from build123d import *

# Parameters (mm, degrees)
BOSS_EXTRUDE23_DEPTH = 1
BOSS_EXTRUDE27_DEPTH = 6
BOSS_EXTRUDE28_START = 6
BOSS_EXTRUDE28_DEPTH = 1
CUT_EXTRUDE9_DEPTH   = 1
SKETCH15_W           = 10
SKETCH15_H           = 2
CUT_EXTRUDE11_DEPTH  = 10
BOSS_EXTRUDE30_DEPTH = 4
BOSS_EXTRUDE31_DEPTH = 3


with BuildPart() as part:
    # Sketch10 → Boss-Extrude23 (new body)
    with BuildSketch(Plane(origin=(0, 0, 0), x_dir=(1, 0, 0), z_dir=(0, 1, 0))):
        with BuildLine():
            Line((-11.5, -13.5), (-10.75, -13.5))
            ThreePointArc((-10.75, -13.5), (-10.603553391, -13.853553391), (-10.25, -14))
            Line((-10.25, -14), (10.25, -14))
            ThreePointArc((10.25, -14), (10.603553391, -13.853553391), (10.75, -13.5))
            Line((10.75, -13.5), (11.5, -13.5))
            Line((11.5, -13.5), (11.5, 13.75))
            ThreePointArc((11.5, 13.75), (11.207106781, 14.457106781), (10.5, 14.75))
            Line((10.5, 14.75), (-10.5, 14.75))
            ThreePointArc((-10.5, 14.75), (-11.207106781, 14.457106781), (-11.5, 13.75))
            Line((-11.5, 13.75), (-11.5, -13.5))
        make_face()
    extrude(amount=BOSS_EXTRUDE23_DEPTH)

    # Sketch10_6 → Boss-Extrude27 (add)
    with BuildSketch(Plane(origin=(0, 0, 0), x_dir=(1, 0, 0), z_dir=(0, 1, 0))):
        with BuildLine():
            Line((-11.5, -13.5), (-10.75, -13.5))
            Line((-10.75, -13.5), (-10.75, 13.5))
            ThreePointArc((-10.75, 13.5), (-10.603553391, 13.853553391), (-10.25, 14))
            Line((-10.25, 14), (10.25, 14))
            ThreePointArc((10.25, 14), (10.603553391, 13.853553391), (10.75, 13.5))
            Line((10.75, 13.5), (10.75, -13.5))
            Line((10.75, -13.5), (11.5, -13.5))
            Line((11.5, -13.5), (11.5, 13.75))
            ThreePointArc((11.5, 13.75), (11.207106781, 14.457106781), (10.5, 14.75))
            Line((10.5, 14.75), (4.75, 14.75))
            Line((4.75, 14.75), (-4.75, 14.75))
            Line((-4.75, 14.75), (-10.5, 14.75))
            ThreePointArc((-10.5, 14.75), (-11.207106781, 14.457106781), (-11.5, 13.75))
            Line((-11.5, 13.75), (-11.5, -13.5))
        make_face()
    extrude(amount=BOSS_EXTRUDE27_DEPTH)

    # Sketch10_7 → Boss-Extrude28 (add)
    with BuildSketch(Plane(origin=(0, 0, 0), x_dir=(1, 0, 0), z_dir=(0, 1, 0)).offset(BOSS_EXTRUDE28_START)):
        with BuildLine():
            Line((-11.5, -13.5), (-10.75, -13.5))
            Line((-10.75, -13.5), (-10.75, 13.5))
            ThreePointArc((-10.75, 13.5), (-10.603553391, 13.853553391), (-10.25, 14))
            Line((-10.25, 14), (10.25, 14))
            ThreePointArc((10.25, 14), (10.603553391, 13.853553391), (10.75, 13.5))
            Line((10.75, 13.5), (10.75, -13.5))
            Line((10.75, -13.5), (11.5, -13.5))
            Line((11.5, -13.5), (11.5, 13.75))
            ThreePointArc((11.5, 13.75), (11.207106781, 14.457106781), (10.5, 14.75))
            Line((10.5, 14.75), (4.75, 14.75))
            Line((4.75, 14.75), (-4.75, 14.75))
            Line((-4.75, 14.75), (-10.5, 14.75))
            ThreePointArc((-10.5, 14.75), (-11.207106781, 14.457106781), (-11.5, 13.75))
            Line((-11.5, 13.75), (-11.5, -13.5))
        make_face()
        with BuildLine():
            Line((10.75, 13.5), (10.75, -13.5))
            ThreePointArc((10.75, -13.5), (10.603553391, -13.853553391), (10.25, -14))
            Line((10.25, -14), (-10.25, -14))
            ThreePointArc((-10.25, -14), (-10.603553391, -13.853553391), (-10.75, -13.5))
            Line((-10.75, -13.5), (-10.75, 13.5))
            ThreePointArc((-10.75, 13.5), (-10.603553391, 13.853553391), (-10.25, 14))
            Line((-10.25, 14), (10.25, 14))
            ThreePointArc((10.25, 14), (10.603553391, 13.853553391), (10.75, 13.5))
        make_face()
    extrude(amount=BOSS_EXTRUDE28_DEPTH)

    # Sketch13 → Cut-Extrude9 (cut)
    with BuildSketch(Plane(origin=(0, 7, 0), x_dir=(1, 0, 0), z_dir=(0, 1, 0))):
        with BuildLine():
            Line((-5, -14), (5, -14))
            ThreePointArc((5, -14), (0, -9), (-5, -14))
        make_face()
    extrude(amount=-CUT_EXTRUDE9_DEPTH, mode=Mode.SUBTRACT)

    # Sketch15 → Cut-Extrude11 (cut)
    with BuildSketch(Plane(origin=(0, 0, -14.75), x_dir=(-1, 0, 0), z_dir=(0, 0, -1))):
        with Locations((0, 2)):
            Rectangle(SKETCH15_W, SKETCH15_H)
    extrude(amount=-CUT_EXTRUDE11_DEPTH, mode=Mode.SUBTRACT)

    # Sketch17 → Boss-Extrude30 (add)
    with BuildSketch(Plane(origin=(0, 7, 0), x_dir=(1, 0, 0), z_dir=(0, 1, 0))):
        with BuildLine():
            Line((-9.25, -6.75), (-9.25, 14.75))
            Line((-9.25, 14.75), (-10, 14.75))
            Line((-10, 14.75), (-10, -7))
            ThreePointArc((-10, -7), (-9.707106781, -7.707106781), (-9, -8))
            Line((-9, -8), (9, -8))
            ThreePointArc((9, -8), (9.707106781, -7.707106781), (10, -7))
            Line((10, -7), (10, 14.75))
            Line((10, 14.75), (9.25, 14.75))
            Line((9.25, 14.75), (9.25, -6.75))
            ThreePointArc((9.25, -6.75), (9.103553391, -7.103553391), (8.75, -7.25))
            Line((8.75, -7.25), (-8.75, -7.25))
            ThreePointArc((-8.75, -7.25), (-9.103553391, -7.103553391), (-9.25, -6.75))
        make_face()
    extrude(amount=BOSS_EXTRUDE30_DEPTH)

    # Sketch18 → Boss-Extrude31 (add)
    with BuildSketch(Plane(origin=(0, 7, 0), x_dir=(1, 0, 0), z_dir=(0, 1, 0))):
        with BuildLine():
            Line((9, 7.5), (9.25, 7.5))
            Line((9.25, 7.5), (9.25, 14.75))
            Line((9.25, 14.75), (8, 14.75))
            Line((8, 14.75), (8, 8.5))
            ThreePointArc((8, 8.5), (8.292893219, 7.792893219), (9, 7.5))
        make_face()
        with BuildLine():
            Line((5, -1.656788855), (0, -1.656788855))
            ThreePointArc((0, -1.656788855), (-0.5, -1.156788855), (0, -0.656788855))
            Line((0, -0.656788855), (5, -0.656788855))
            ThreePointArc((5, -0.656788855), (5.5, -1.156788855), (5, -1.656788855))
        make_face()
        with BuildLine():
            Line((-9.25, 7.5), (-9, 7.5))
            ThreePointArc((-9, 7.5), (-8.292893219, 7.792893219), (-8, 8.5))
            Line((-8, 8.5), (-8, 14.75))
            Line((-8, 14.75), (-9.25, 14.75))
            Line((-9.25, 14.75), (-9.25, 7.5))
        make_face()
    extrude(amount=BOSS_EXTRUDE31_DEPTH)


solid = part.part
Read the model definition and answer for the solid it produces. Units are mm, in the model's axes. A direction names the side the tool comes from. Coordinates: 2 decimals unless noted, no trailing zeros. Loops run counter-clockwise (first coordinate to the right, second up) from the corner with the lowest first, then second, coordinate; pieces in that order, holes last. Notation, with made-up numbers: (-12, -27.75) -> (7, -27.75) arc R24 cw to (7, 10.25) -> close; hole circle Ø10 at (67.25, -8). An arc over 180 degrees is marked (long way). Write item = value, one per line. Start each with the question number.
1) Given P1, Ø1, axis at x = -8.5, z = -10.5, coming from the +Y side; P2, Ø4, axis at x = 2.5, y = 4.5, coming from the +Z side; P3, Ø1.5, axis at x = 1.5, y = 9, coming from the -Z side, each flat-ended and moving along its own axis, determine where each tip first touches the part or whether it passes through.
2) Find the intervals of material crossed by L1, parallel to X at y = 3.25, z = -11; L2, parallel to Y at x = 8.5, z = -2.5; L3, parallel to Z at x = 1.5, y = 7.75, in increasing order. Write a range as from..to.
3) The part is cut by section C-C, the plane y = 5.25. Determine the outline of the cut face in (x, z).
4) The mould has two halves that part along Y. Classify faces 1 (the face through (-8.301, 8.479, -7.785)), 2 (the face through (-10.75, 3, 0)), 3 (the face through (-9, 10, -11)): pulls with the +Y half, pulls with the -Y half, needs draft (parallel to the pull), parting line crosses it, or undercut.
5) The part is cut by section A-A, the plane x = 6.25. Determine the outline of the cut face in (y, z).
6) For faces 4 (the face through (9, 10, -11)), 5 (the face through (9.25, 9, -2)), 6 (the face through (0, 9, 8)), determine the directions among +Z, -Z, +X, -X, +Y, -Y from which every point of the face is accessible in a straight line to the end or side of a thin tool.
7) The part is cut by section D-D, the plane x = -4.5. Determine the outline of the cut face in (y, z).
8) The part is cut by section B-B, the plane z = -11.25. Determine the outline of the cut face in (x, y).
Result:
q1.P1 = 10
q1.P2 = 10.78
q1.P3 = 0.66
q2.L1 = -11.5..-10.75, 10.75..11.5
q2.L2 = 0..1, 6..7
q2.L3 = 0.66..1.66, 7.25..8
q3.outline = (-11.5, -13.75) arc R1 ccw to (-10.5, -14.75) -> (10.5, -14.75) arc R1 ccw to (11.5, -13.75) -> (11.5, 13.5) -> (10.75, 13.5) -> (10.75, -13.5) arc R0.5 cw to (10.25, -14) -> (-10.25, -14) arc R0.5 cw to (-10.75, -13.5) -> (-10.75, 13.5) -> (-11.5, 13.5) -> close
q4.face_1 = needs draft
q4.face_2 = undercut
q4.face_3 = pulls with the +Y half
q5.outline = (0, -14.75) -> (7, -14.75) -> (7, 7.25) -> (11, 7.25) -> (11, 8) -> (7, 8) -> (7, 14) -> (6, 14) -> (6, -14) -> (1, -14) -> (1, 14) -> (0, 14) -> close
q6.face_4 = -Z, +Y
q6.face_5 = +Y
q6.face_6 = +Z, +X, -X, +Y
q7.outline = (0, -14.75) -> (1, -14.75) -> (1, 14) -> (0, 14) -> close; (3, -14.75) -> (7, -14.75) -> (7, 7.25) -> (11, 7.25) -> (11, 8) -> (7, 8) -> (7, 11.82) -> (6, 11.82) -> (6, -14) -> (3, -14) -> close
q8.outline = (-11.5, 0) -> (11.5, 0) -> (11.5, 7) -> (10, 7) -> (10, 11) -> (9.25, 11) -> (9.25, 10) -> (8, 10) -> (8, 7) -> (-8, 7) -> (-8, 10) -> (-9.25, 10) -> (-9.25, 11) -> (-10, 11) -> (-10, 7) -> (-11.5, 7) -> close; hole (-10.75, 1) -> (10.75, 1) -> (10.75, 6) -> (-10.75, 6) -> close
